```python
from build123d import *

# Parameters (mm, degrees)
SKETCH_1_R               = 13
EXTRUDE_1_DEPTH          = 3.7
SKETCH_3_R               = 2.4
SKETCH_3_R_2             = 0.5
EXTRUDE_3_DEPTH          = 7.9
PATTERN_CIRCULAR_1_COUNT = 6
SKETCH_4_R               = 0.9
CUT_EXTRUDE_1_DEPTH      = 21.010247375
PATTERN_CIRCULAR_2_COUNT = 3
SKETCH_5_R               = 1.1
CUT_EXTRUDE_2_DEPTH      = 21.010247375
SKETCH_5_4_R             = 2.55
SKETCH_5_4_R_2           = 1.1
CUT_EXTRUDE_3_DEPTH      = 2.6


with BuildPart() as part:
    # Sketch 1 → Extrude 1 (new body)
    with BuildSketch(Plane.XY):
        Circle(SKETCH_1_R)
    extrude(amount=EXTRUDE_1_DEPTH)

    # Sketch 3 → Extrude 3 (add)
    with BuildSketch(Plane.XY.offset(3.7)):
        with Locations((-5.656854249, 5.656854249)):
            Circle(SKETCH_3_R)
        with Locations((-5.656854249, 5.656854249)):
            Circle(SKETCH_3_R_2, mode=Mode.SUBTRACT)
    extrude_3 = extrude(amount=EXTRUDE_3_DEPTH)

    # Pattern Circular 1: Extrude 3 ×6 about axis
    pattern_circular_1_axis = Axis((0, 0, 0), (0, 0, 1))
    for i in range(1, PATTERN_CIRCULAR_1_COUNT):
        add(extrude_3.rotate(pattern_circular_1_axis, i * 360 / PATTERN_CIRCULAR_1_COUNT))

    # Sketch 4 → Cut-Extrude 1 (cut, through all)
    with BuildSketch(Plane.XY.offset(3.7)):
        with Locations((-2.588190451, 9.659258263)):
            Circle(SKETCH_4_R)
    cut_extrude_1 = extrude(amount=-CUT_EXTRUDE_1_DEPTH, mode=Mode.SUBTRACT)

    # Pattern Circular 2: Cut-Extrude 1 ×3 about axis
    pattern_circular_2_axis = Axis((0, 0, 0), (0, 0, 1))
    for i in range(1, PATTERN_CIRCULAR_2_COUNT):
        add(cut_extrude_1.rotate(pattern_circular_2_axis, i * 360 / PATTERN_CIRCULAR_2_COUNT), mode=Mode.SUBTRACT)

    # Sketch 5 → Cut-Extrude 2 (cut, through all)
    with BuildSketch(Plane.XY.offset(3.7)):
        Circle(SKETCH_5_R)
    extrude(amount=-CUT_EXTRUDE_2_DEPTH, mode=Mode.SUBTRACT)

    # Sketch 5_4 → Cut-Extrude 3 (cut)
    with BuildSketch(Plane.XY.offset(3.7)):
        Circle(SKETCH_5_4_R)
        Circle(SKETCH_5_4_R_2, mode=Mode.SUBTRACT)
    extrude(amount=-CUT_EXTRUDE_3_DEPTH, mode=Mode.SUBTRACT)


solid = part.part
```
Build history of the part. All positions in model axes, mm. A direction names the side the tool comes from. Coordinates: 2 decimals unless noted, no trailing zeros. Order: outer loops, then holes, each group sorted by start corner. A loop starts at its lowest first (then second) coordinate and runs counter-clockwise, first axis right, second up. Notation, with made-up numbers: (50.5, 64.5) -> (55.5, 64.5) arc R16 cw to (55.5, 80.5) -> close; hole circle Ø8 at (41, -36.5). An arc over 180 degrees is marked (long way). Answer in a Markdown table with one row per item. Add a question column.
Q1. Band-saw the part on C-C, the plane x = -9.75. List the corners of the cut face in (y, z), then the cut area to 3 significant figures.
Q2. Which spindle directions (+Z, -Z, +X, -X, +Y, -Y) get a long thin tool onto all of the face, cutting with end or side? Do faces 1 (the face through (-5.39, 6.08, 7.59)), 2 (the face through (-2.173, 8.861, 1.876)). Say none if no direction does.
Q3. Band-saw the part on A-A, the plane z = 7.25. Give the number of separate pieces and of enclosed holes in the cut face, then the cut area to 3 significant figures.
Q4. Wall check: line 1 along Y through (x, z) = (0, 0.5); line 2 along Y through (x, z) = (-6, 8); line 3 along Z through (x, y) = (-5.75, -10.75). Give the ranges that are in metal, low to high. Write a range as [from, to].
Q5. Drop flat-ended pins along their axis: pin 1 (6 mm diameter, centred on x = 0, y = 0, fed in from +Z); pin 2 (2.5 mm diameter, centred on x = 0, y = 0, fed in from +Z); pin 3 (1 mm diameter, centred on y = -6.5, z = 5, fed in from +X). Give the stop position or say it passes through.
Q6. Mould opens along X. For faces 3 (the face through (-10.316, -7.91, 1.824)), 4 (the face through (6.177, -3.314, 7.595)), 5 (the face through (3, 0, 3.7)), 6 (the face through (-7, -2, 11.6)) say: +X half, -X half, draft (parallel to the pull), parting line (faces both ways), or undercut.
Q7. Band-saw the part on B-B, the plane x = 0. List the corners of the cut face in (y, z).
Answers follow:
| question | item | result |
|---|---|---|
| 1 | outline | (-8.6, 0) -> (8.6, 0) -> (8.6, 3.7) -> (-0.78, 3.7) -> (-0.78, 11.6) -> (-3.36, 11.6) -> (-3.36, 3.7) -> (-8.6, 3.7) -> close |
| 1 | area | 84.0 mm^2 |
| 2 | face 1 | +Z |
| 2 | face 2 | +Z, -Z |
| 3 | separate pieces | 6 |
| 3 | enclosed holes | 6 |
| 3 | area | 104 mm^2 |
| 4 | line 1 | [-13, -1.1], [1.1, 13] |
| 4 | line 2 | [-3.74, -0.4], [3.28, 5.29], [6.02, 8.03] |
| 4 | line 3 | [0, 3.7] |
| 5 | pin 1 | z = 3.7 |
| 5 | pin 2 | z = 1.1 |
| 5 | pin 3 | x = 8.03 |
| 6 | face 3 | parting line |
| 6 | face 4 | undercut |
| 6 | face 5 | undercut |
| 6 | face 6 | draft |
| 7 | outline | (-13, 0) -> (-1.1, 0) -> (-1.1, 1.1) -> (-2.55, 1.1) -> (-2.55, 3.7) -> (-6.51, 3.7) -> (-6.51, 11.6) -> (-8.94, 11.6) -> (-8.94, 3.7) -> (-13, 3.7) -> close; (1.1, 0) -> (13, 0) -> (13, 3.7) -> (8.94, 3.7) -> (8.94, 11.6) -> (6.51, 11.6) -> (6.51, 3.7) -> (2.55, 3.7) -> (2.55, 1.1) -> (1.1, 1.1) -> close |
